Here's how the part is built. I have some questions about the finished solid (model axes, mm). Face numbers are marked on the shaded views. A direction names the side the tool comes from. Give positions to 0.01 mm unless a question says otherwise; leave off trailing zeros. Order: outer loops, then holes, each group sorted by start corner. A loop starts at its lowest first (then second) coordinate and runs counter-clockwise, first axis right, second up.
from build123d import *

# Parameters (mm, degrees)
SKETCH1_W            = 20
SKETCH1_H            = 25
BOSS_EXTRUDE1_DEPTH  = 2
SKETCH2_W            = 20
SKETCH2_H            = 12.7
BOSS_EXTRUDE2_DEPTH  = 3
M3_CLEARANCE_HOLE1_D = 3.4
SKETCH7_R            = 9
CUT_EXTRUDE1_DEPTH   = 20.856296231
SKETCH8_W            = 20
SKETCH8_H            = 5.35
CUT_EXTRUDE2_DEPTH   = 28.910974544


with BuildPart() as part:
    # Sketch1 → Boss-Extrude1 (new body)
    with BuildSketch(Plane.XY):
        Rectangle(SKETCH1_W, SKETCH1_H)
    extrude(amount=BOSS_EXTRUDE1_DEPTH)

    # Sketch2 → Boss-Extrude2 (add)
    with BuildSketch(Plane.XZ.offset(12.5)):
        with Locations((0, 1)):
            Rectangle(SKETCH2_W, SKETCH2_H)
    extrude(amount=BOSS_EXTRUDE2_DEPTH)

    # M3 Clearance Hole1 (through all)
    with Locations(Plane(origin=(0, -12.5, 0), x_dir=(1, 0, 0), z_dir=(0, 1, 0))):
        with Locations((-5.715, 2.739497088), (5.715, 2.739497088)):
            Hole(M3_CLEARANCE_HOLE1_D / 2)

    # Sketch7 → Cut-Extrude1 (cut, through all)
    with BuildSketch(Plane.XY.offset(2)):
        with Locations((0, 0.5)):
            Circle(SKETCH7_R)
    extrude(amount=-CUT_EXTRUDE1_DEPTH, mode=Mode.SUBTRACT)

    # Sketch8 → Cut-Extrude2 (cut, through all)
    with BuildSketch(Plane(origin=(0, -12.5, 0), x_dir=(1, 0, 0), z_dir=(0, 1, 0))):
        with Locations((0, -4.675)):
            Rectangle(SKETCH8_W, SKETCH8_H)
    extrude(amount=-CUT_EXTRUDE2_DEPTH, mode=Mode.SUBTRACT)


solid = part.part
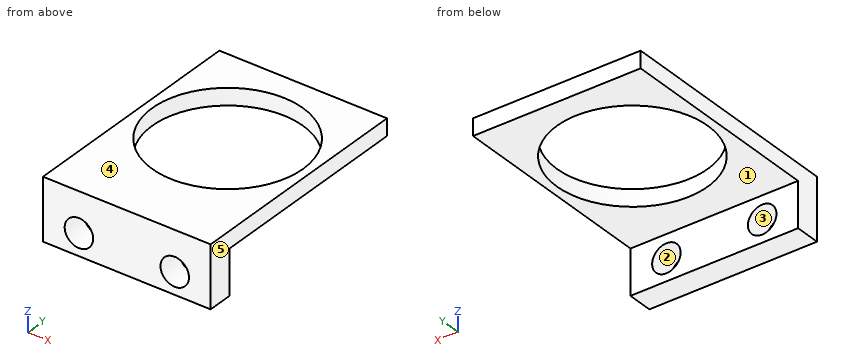
Q1. If we section it at D-D on x = 6: List the corners of the cut face in (y, z) for me.
Filled sheet:
outline: (-15.5, -5.35) - (-12.5, -5.35) - (-12.5, -4.42) - (-15.5, -4.42) - close; (-15.5, -1.06) - (-12.5, -1.06) - (-12.5, 0) - (-6.21, 0) - (-6.21, 2) - (-15.5, 2) - close; (7.21, 0) - (12.5, 0) - (12.5, 2) - (7.21, 2) - close
Q2. I need wall thicknesses on L1, parallel to Y at x = 0, z = 1.4; L2, parallel to Y at x = 7.5, z = -2.25; L3, parallel to Z at x = -0.75, y = -11. Which ranges of each line are inside material? Lowest first, please.
Filled sheet:
L1: y = -15.5 to -8.5, 9.5 to 12.5
L2: y = -15.5 to -12.5
L3: z = 0 to 2
Q3. If we section it at C-C on z = 0.75: List the corners of the cut face in (x, y) for me, plus the area to 3 significant figures.
Filled sheet:
outline: (-10, -15.5) - (10, -15.5) - (10, 12.5) - (-10, 12.5) - close; hole circle Ø18 at (0, 0.5)
area: 306 mm2
Q4. I'm going to push flat-ended pins straight in: P1, Ø6, axis at x = -0.5, y = -7.5, coming from the -Z side; P2, Ø2.5, axis at x = -3, z = -4, coming from the +Y side; P3, Ø3, axis at y = 4.5, z = -1, coming from the +X side. Where does each tip first touch, or does it pass through?
Filled sheet:
P1: stops at z = 0
P2: stops at y = -12.5
P3: stops at x = 10
Q5. If we section it at A-A on x = 0: List the corners of the cut face in (y, z) for me.
Filled sheet:
outline: (-15.5, -5.35) - (-12.5, -5.35) - (-12.5, 0) - (-8.5, 0) - (-8.5, 2) - (-15.5, 2) - close; (9.5, 0) - (12.5, 0) - (12.5, 2) - (9.5, 2) - close
Q6. For the marked faces 1 and 2, which set-ups out of +Z, -Z, +X, -X, +Y, -Y let a thin tool reach every point of the face, with its end or its side?
Filled sheet:
face 1: -Z, +X, -X, +Y
face 2: +Y, -Y
Q7. Thinking about a two-plate mould opening in X: for the marked faces 3, 4 and 5, which applies, released by +X, released by -X, zero draft, split by the parting line, or undercut?
Filled sheet:
face 3: undercut
face 4: zero draft
face 5: released by +X
Q8. If we section it at B-B on y = 0.5: List the corners of the cut face in (x, z) for me.
Filled sheet:
outline: (-10, 0) - (-9, 0) - (-9, 2) - (-10, 2) - close; (9, 0) - (10, 0) - (10, 2) - (9, 2) - close
